```python
from build123d import *

# Parameters (mm, degrees)
SKETCH1_W           = 44.45
SKETCH1_H           = 31.75
BOSS_EXTRUDE1_DEPTH = 3.175
SKETCH2_R           = 2.2225
SKETCH2_R_2         = 1.143
BOSS_EXTRUDE2_DEPTH = 10.16
SKETCH3_R           = 1.7145
CUT_EXTRUDE1_DEPTH  = 12.7
SKETCH4_R           = 1.7145
CUT_EXTRUDE2_DEPTH  = 12.7
CIRPATTERN1_COUNT   = 4
FILLET1_R           = 2.032


with BuildPart() as part:
    # Sketch1 → Boss-Extrude1 (new body)
    with BuildSketch(Plane.XY):
        with Locations((-22.225, -15.875)):
            Rectangle(SKETCH1_W, SKETCH1_H)
    extrude(amount=BOSS_EXTRUDE1_DEPTH)

    # Sketch2 → Boss-Extrude2 (add)
    with BuildSketch(Plane.XY.offset(3.175)):
        with Locations((-41.91, -2.54)):
            Circle(SKETCH2_R)
        with Locations((-41.91, -2.54)):
            Circle(SKETCH2_R_2, mode=Mode.SUBTRACT)
        with Locations((-25.4, -17.145)):
            Circle(SKETCH2_R)
        with Locations((-25.4, -17.145)):
            Circle(SKETCH2_R_2, mode=Mode.SUBTRACT)
    extrude(amount=BOSS_EXTRUDE2_DEPTH)

    # Sketch3 → Cut-Extrude1 (cut)
    with BuildSketch(Plane.XY.offset(3.175)):
        with Locations((-7.62, -3.175)):
            Circle(SKETCH3_R)
        with Locations((-7.62, -28.575)):
            Circle(SKETCH3_R)
    extrude(amount=-CUT_EXTRUDE1_DEPTH, mode=Mode.SUBTRACT)

    # Sketch4 → Cut-Extrude2 (cut)
    with BuildSketch(Plane.XY.offset(3.175)):
        with Locations((-25.4, -7.366)):
            Circle(SKETCH4_R)
    cut_extrude2 = extrude(amount=-CUT_EXTRUDE2_DEPTH, mode=Mode.SUBTRACT)

    # CirPattern1: Cut-Extrude2 ×4 about axis
    cirpattern1_axis = Axis((-25.4, -17.145, 0), (0, 0, 1))
    for i in range(1, CIRPATTERN1_COUNT):
        add(cut_extrude2.rotate(cirpattern1_axis, i * 360 / CIRPATTERN1_COUNT), mode=Mode.SUBTRACT)

    # Fillet1
    fillet1_edges = [part.edges().sort_by_distance(p)[0] for p in [
        (0, -31.75, 1.5875),
        (-44.45, -31.75, 1.5875),
        (-44.45, 0, 1.5875),
        (0, 0, 1.5875),
    ]]
    fillet(fillet1_edges, radius=FILLET1_R)


solid = part.part
```
The model under review builds one solid part; all positions refer to its coordinate system, in mm. A direction names the side the tool comes from. Round coordinates to 2 decimals unless told otherwise and drop trailing zeros. Use a Markdown table: item, result. Add a question column.
Q1. For probe 1 along Y at (x, z) = (-25.4, 1.15); probe 2 along Z at (x, y) = (-15.5, -22) (3 decimals); probe 3 along X at (y, z) = (-3, 10.75), list the stretches that pass through material, from the lowest coordinate up.
Q2. Machinability: for faces 4 (the face through (-40.82, -2.2, 8.18)), 5 (the face through (-0.61, -0.58, 1.61)), which of the approach directions +Z, -Z, +X, -X, +Y, -Y give a long, thin tool a straight path to every point of the face, cutting with its end or side? Answer none if there is none.
Q3. Add section A-A (x = -7.62). State how many separate pieces and enclosed holes the cut face has, plus the area to 3 significant figures.
Q4. Insertion check: pin 1 Ø1.5 at (x, y) = (-35, -6.5) entering from +Z (3 decimals); pin 2 Ø8 at (x, y) = (-39, -20) entering from -Z. Each pin has a flat end and moves straight along its axis. Give the tip position at first contact, or say it passes through.
Q5. The part is to be moulded in two halves that separate along Y. For faces 1 (the face through (-24.04, -25.88, 1.61)), 2 (the face through (-27.16, -18.5, 8.18)), 3 (the face through (-23, -31.75, 2)), say which applies: pulls with the +Y half, pulls with the -Y half, needs draft (parallel to the pull), parting line crosses it, or undercut.
Worked answers:
| question | item | result |
|---|---|---|
| 1 | probe 1 | -31.75 to -28.64, -25.21 to -9.08, -5.65 to 0 |
| 1 | probe 2 | 0 to 3.175 |
| 1 | probe 3 | -44.08 to -42.96, -40.86 to -39.74 |
| 2 | face 4 | +Z |
| 2 | face 5 | +Z, -Z, +X, +Y |
| 3 | separate pieces | 3 |
| 3 | enclosed holes | 0 |
| 3 | area | 79.0 mm² |
| 4 | pin 1 | z = 3.175 |
| 4 | pin 2 | z = 0 |
| 5 | face 1 | undercut |
| 5 | face 2 | parting line crosses it |
| 5 | face 3 | pulls with the -Y half |
